For this review, take the finished solid that the model builds, in its own axes (mm). Face numbers are marked on the shaded views. A direction names the side the tool comes from. Give positions to 0.01 mm unless a question says otherwise; leave off trailing zeros. Loops run counter-clockwise (first coordinate to the right, second up) from the corner with the lowest first, then second, coordinate; pieces in that order, holes last. Notation, with made-up numbers: (19.5, -28.75) -> (36.5, -28.75) arc R29 cw to (36.5, 2.25) -> close; hole circle Ø10 at (48, -34.5). An arc over 180 degrees is marked (long way). Write each question's results on one line, items separated by ' | '. Start each with the question number.
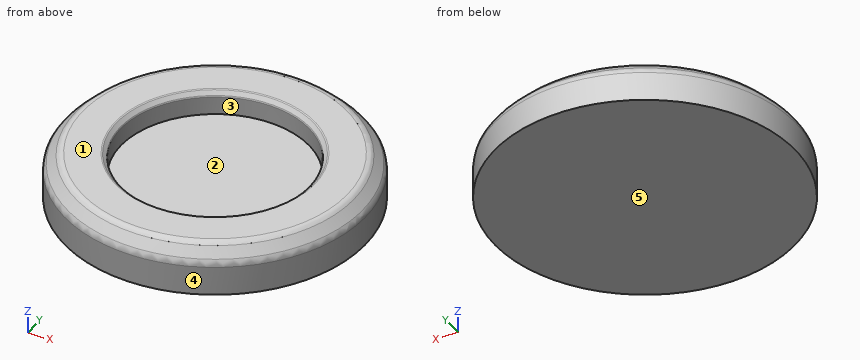
```python
from build123d import *

# Parameters (mm, degrees)
SKETCH1_R           = 31.93
BOSS_EXTRUDE1_DEPTH = 10
CHAMFER1_SIZE       = 3
FILLET1_R           = 2
SKETCH2_R           = 20
CUT_EXTRUDE1_DEPTH  = 5
CHAMFER2_SIZE       = 1
FILLET2_R           = 0.4


with BuildPart() as part:
    # Sketch1 → Boss-Extrude1 (new body)
    with BuildSketch(Plane.XY):
        Circle(SKETCH1_R)
    extrude(amount=BOSS_EXTRUDE1_DEPTH)

    # Chamfer1
    chamfer1_edges = [part.edges().sort_by_distance(p)[0] for p in [
        (-31.93, 0, 10),
    ]]
    chamfer(chamfer1_edges, length=CHAMFER1_SIZE)

    # Fillet1
    fillet1_edges = [part.edges().sort_by_distance(p)[0] for p in [
        (-28.93, 0, 10),
        (-31.93, 0, 7),
    ]]
    fillet(fillet1_edges, radius=FILLET1_R)

    # Sketch2 → Cut-Extrude1 (cut)
    with BuildSketch(Plane.XY.offset(10)):
        Circle(SKETCH2_R)
    extrude(amount=-CUT_EXTRUDE1_DEPTH, mode=Mode.SUBTRACT)

    # Chamfer2
    chamfer2_edges = [part.edges().sort_by_distance(p)[0] for p in [
        (-20, 0, 10),
    ]]
    chamfer(chamfer2_edges, length=CHAMFER2_SIZE)

    # Fillet2
    fillet2_edges = [part.edges().sort_by_distance(p)[0] for p in [
        (-20, 0, 9),
        (-21, 0, 10),
    ]]
    fillet(fillet2_edges, radius=FILLET2_R)


solid = part.part
```
1. Draft analysis for pull direction Y (two halves, no side actions). For the marked faces 3, 4 and 5, state which applies: released by +Y, released by -Y, zero draft, split by the parting line, or undercut.
2. Wall thickness on L1, parallel to Y at x = 0, z = 6; L2, parallel to Z at x = 13.5, y = 5: over which ranges is each line inside the solid? List them lowest first.
3. We need section A-A (z = 2.75). Write out the cut boundary in (x, y), plus the area to 3 significant figures.
4. Machinability: for the marked faces 1 and 2, which of the approach directions +Z, -Z, +X, -X, +Y, -Y give a long, thin tool a straight path to every point of the face, cutting with its end or side? Answer none if there is none.
5. For pin 1 Ø6 at (y, z) = (25, 6) entering from +X; pin 2 Ø4 at (y, z) = (23, 6.5) entering from +X; pin 3 Ø1 at (y, z) = (-24, 7) entering from +X, all flat-tipped, find the tip position at first contact; note any pin that passes through.
Response:
1) face 3: undercut | face 4: split by the parting line | face 5: zero draft
2) L1: y = -31.93 to -20, 20 to 31.93 | L2: z = 0 to 5
3) outline: circle Ø63.86 at (0, 0) | area: 3,200 mm2
4) face 1: +Z, +X, -X, +Y, -Y | face 2: +Z
5) pin 1: stops at x = 23.14 | pin 2: stops at x = 24.04 | pin 3: stops at x = 21.42
